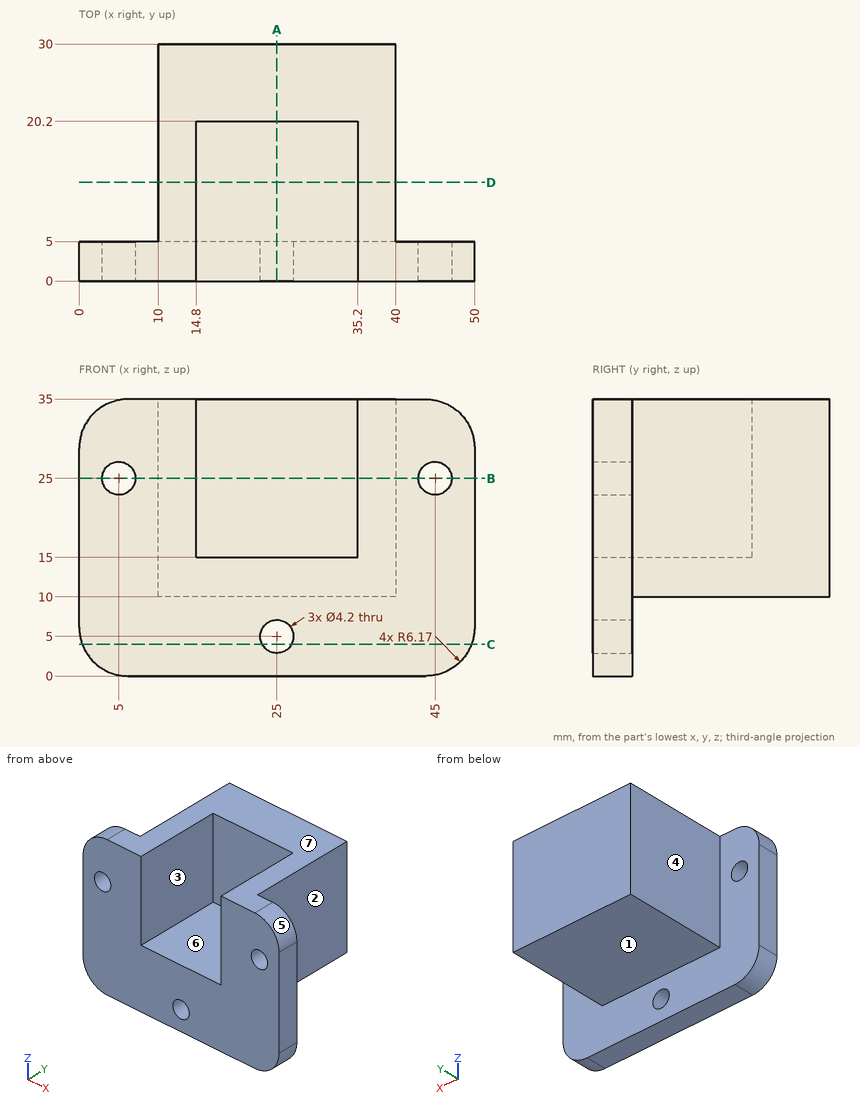
Here's the drawing with two shaded views (mm, measured from the low corner). I have some questions. A direction names the side the tool comes from. Give positions to 0.01 mm unless a question says otherwise; leave off trailing zeros. Order: outer loops, then holes, each group sorted by start corner. A loop starts at its lowest first (then second) coordinate and runs counter-clockwise, first axis right, second up. Notation, with made-up numbers: (1, 68) -> (20, 68) arc R35 cw to (20, 100) -> close; hole circle Ø1 at (48.5, -1). An arc over 180 degrees is marked (long way). Use a Markdown table: item, result. Add a question column.
Item 1: Will these pins go through, and if not, where does the flat tip stop? pin 1 (8 mm diameter, centred on x = 10, y = 21, fed in from -Z); pin 2 (12 mm diameter, centred on y = 22.5, z = 11, fed in from +X); pin 3 (3.5 mm diameter, centred on x = 25, z = 5, fed in from -Y); pin 4 (6.5 mm diameter, centred on x = 45, z = 25, fed in from +Y).
Item 2: Imagine slicing it at A-A on x = 25. Please give me the cut outline in (y, z), plus the area to 3 significant figures.
Item 3: If we mould it in two halves opening along X, with no side actions, what happens to the marked faces 5, 6 and 7? For each: pulls with the +X half, pulls with the -X half, needs draft (parallel to the pull), parting line crosses it, or undercut.
Item 4: Imagine slicing it at D-D on y = 12.5. Please give me the cut outline in (x, z).
Item 5: I need wall thicknesses on line 1 (X direction, y = 1.5, z = 25); line 2 (Z direction, x = 25, y = 1.45); line 3 (X direction, y = 4.75, z = 22). Which ranges of each line are inside material? Lowest first, please.
Item 6: Imagine slicing it at B-B on z = 25. Please give me the cut outline in (x, y).
Item 7: Imagine slicing it at C-C on z = 4. Please give me the cut outline in (x, y).
Item 8: For the marked faces 1, 2, 3 and 4, which set-ups out of +Z, -Z, +X, -X, +Y, -Y let a thin tool reach every point of the face, with its end or its side?
Data:
| question | item | result |
|---|---|---|
| 1 | pin 1 | stops at z = 10 |
| 1 | pin 2 | stops at x = 40 |
| 1 | pin 3 | passes through |
| 1 | pin 4 | stops at y = 5 |
| 2 | outline | (0, 0) -> (5, 0) -> (5, 2.9) -> (0, 2.9) -> close; (0, 7.1) -> (5, 7.1) -> (5, 10) -> (30, 10) -> (30, 35) -> (20.2, 35) -> (20.2, 15) -> (0, 15) -> close |
| 2 | area | 375 mm² |
| 3 | face 5 | pulls with the +X half |
| 3 | face 6 | undercut |
| 3 | face 7 | needs draft |
| 4 | outline | (10, 10) -> (40, 10) -> (40, 35) -> (35.2, 35) -> (35.2, 15) -> (14.8, 15) -> (14.8, 35) -> (10, 35) -> close |
| 5 | line 1 | x = 0 to 2.9, 7.1 to 14.8, 35.2 to 42.9, 47.1 to 50 |
| 5 | line 2 | z = 0 to 2.9, 7.1 to 15 |
| 5 | line 3 | x = 0 to 14.8, 35.2 to 50 |
| 6 | outline | (0, 0) -> (2.9, 0) -> (2.9, 5) -> (0, 5) -> close; (7.1, 0) -> (14.8, 0) -> (14.8, 20.2) -> (35.2, 20.2) -> (35.2, 0) -> (42.9, 0) -> (42.9, 5) -> (40, 5) -> (40, 30) -> (10, 30) -> (10, 5) -> (7.1, 5) -> close; (47.1, 0) -> (50, 0) -> (50, 5) -> (47.1, 5) -> close |
| 7 | outline | (0.39, 0) -> (23.15, 0) -> (23.15, 5) -> (0.39, 5) -> close; (26.85, 0) -> (49.61, 0) -> (49.61, 5) -> (26.85, 5) -> close |
| 8 | face 1 | -Z, +X, -X, +Y |
| 8 | face 2 | +Z, -Z, +X, +Y |
| 8 | face 3 | +Z, -Y |
| 8 | face 4 | +Z, -Z, -X, +Y |
